Design review of the part shown in the three views and the two pictorial views. Dimensions are in mm from the part's minimum x, y and z. Coordinates: 2 decimals unless noted, no trailing zeros. Order: outer loops, then holes, each group sorted by start corner. A loop starts at its lowest first (then second) coordinate and runs counter-clockwise, first axis right, second up. Notation, with made-up numbers: M 78,-34.5 L 131,-34.5 A13 ccw 131,-26.5 Z; hole C 55.5,78.25 d4. An arc over 180 degrees is marked long. Use CSV: the item, a comma, the result in double quotes.
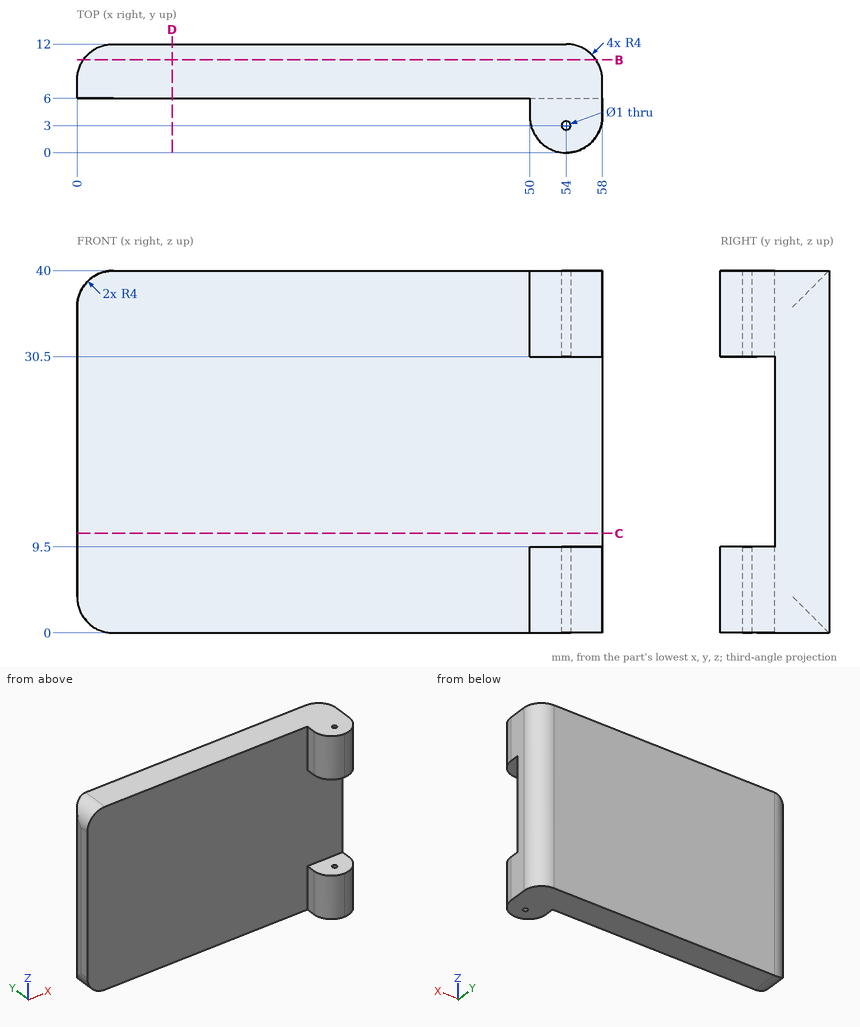
(1) Add section B-B on y = 10.25. State the section outline as (x, z) points.
The answers:
outline,"M 0.69,1.75 A4 ccw 4,0 L 57.31,0 L 57.31,40 L 4,40 A4 ccw 0.69,38.25 Z"
(2) Add section D-D on x = 10.5. State the section outline as (y, z) points.
The answers:
outline,"M 6,0 L 12,0 L 12,40 L 6,40 Z"
(3) Clearance check with flat-ended pins moving along their axes: P1, Ø5, axis at x = 32, z = 4.5, coming from the -Y side; P2, Ø0.6, axis at y = 4.5, z = 6.5, coming from the -X side; P3, Ø1.5, axis at y = 9, z = 8.5, coming from the -X side. State where each tip first meets the part, or that it passes through.
The answers:
P1,"stops at y = 6"
P2,"stops at x = 50"
P3,"stops at x = 0.01"
(4) Wall thickness on probe 1 along Y at (x, z) = (54, 34); probe 2 along Y at (x, z) = (53, 12.5); probe 3 along X at (y, z) = (3.75, 33.5): over which ranges is each line inside the solid? List them lowest first.
The answers:
probe 1,"y = 0 to 2.5, 3.5 to 12"
probe 2,"y = 6 to 12"
probe 3,"x = 50.01 to 57.99"
(5) Add section C-C on z = 11. State the section outline as (x, y) points.
The answers:
outline,"M 0,6 L 58,6 L 58,8 A4 ccw 54,12 L 4,12 A4 ccw 0,8 Z"
